Part print with two shaded views. Sizes in mm from the minimum x, y, z corner. Round coordinates to 2 decimals unless told otherwise and drop trailing zeros. Loops run counter-clockwise (first coordinate to the right, second up) from the corner with the lowest first, then second, coordinate; pieces in that order, holes last.
(1) Flat gauge pins, fed straight in: pin 1 (3 mm diameter, centred on x = 275, y = 145, fed in from -Z); pin 2 (3 mm diameter, centred on x = 7, z = 4, fed in from +Y); pin 3 (3 mm diameter, centred on y = 4.5, z = 2.5, fed in from +X). Where does each tip first touch, or does it go through?
(2) Cut at A-A on x = 140. List the corners of the cut face in (y, z), then the cut area to 3 significant figures.
(3) Cut at B-B on z = 4.25. Count the separate pieces of the cut face and the enclosed holes in it, then the cut area to 3 significant figures.
(4) Probe probe 1 along Y at (x, z) = (124.5, 2.6); probe 2 along X at (y, z) = (36.65, 1.9); probe 3 along Y at (x, z) = (5, 4.5). List the from-to ranges inside material, lowest first.
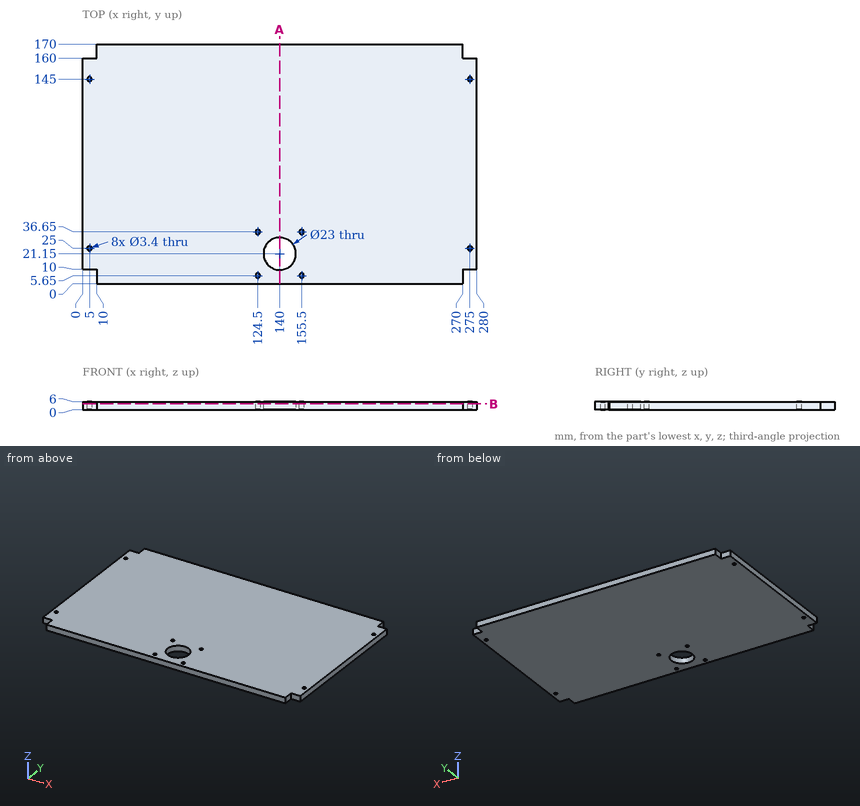
Final values:
1. pin 1: passes through
1. pin 2: stops at y = 160
1. pin 3: stops at x = 270
2. outline: (0, 0) - (9.65, 0) - (9.65, 6) - (0, 6) - close; (32.65, 0) - (170, 0) - (170, 6) - (32.65, 6) - close
2. area: 882 mm2
3. separate pieces: 1
3. enclosed holes: 9
3. area: 46,700 mm2
4. probe 1: y = 0 to 3.95, 7.35 to 34.95, 38.35 to 170
4. probe 2: x = 0 to 122.8, 126.2 to 153.8, 157.2 to 280
4. probe 3: y = 10 to 23.3, 26.7 to 143.3, 146.7 to 160
